Input: dimensioned drawing with shaded views. Units: mm. Origin: part minimum x, y, z. A direction names the side the tool comes from. Give positions to 0.01 mm unless a question says otherwise; leave off trailing zeros. Write each loop counter-clockwise with the first axis right and the second up, starting at its lowest first coordinate (ties: lowest second). Pieces come first, ordered by that corner, then holes. Notation, with made-up numbers: (3.25, -33) - (22.25, -33) arc R25 ccw to (22.25, 5) - close; hole circle Ø11 at (89, -4). An arc over 180 degrees is marked (long way). Answer as CSV lines item,"result".
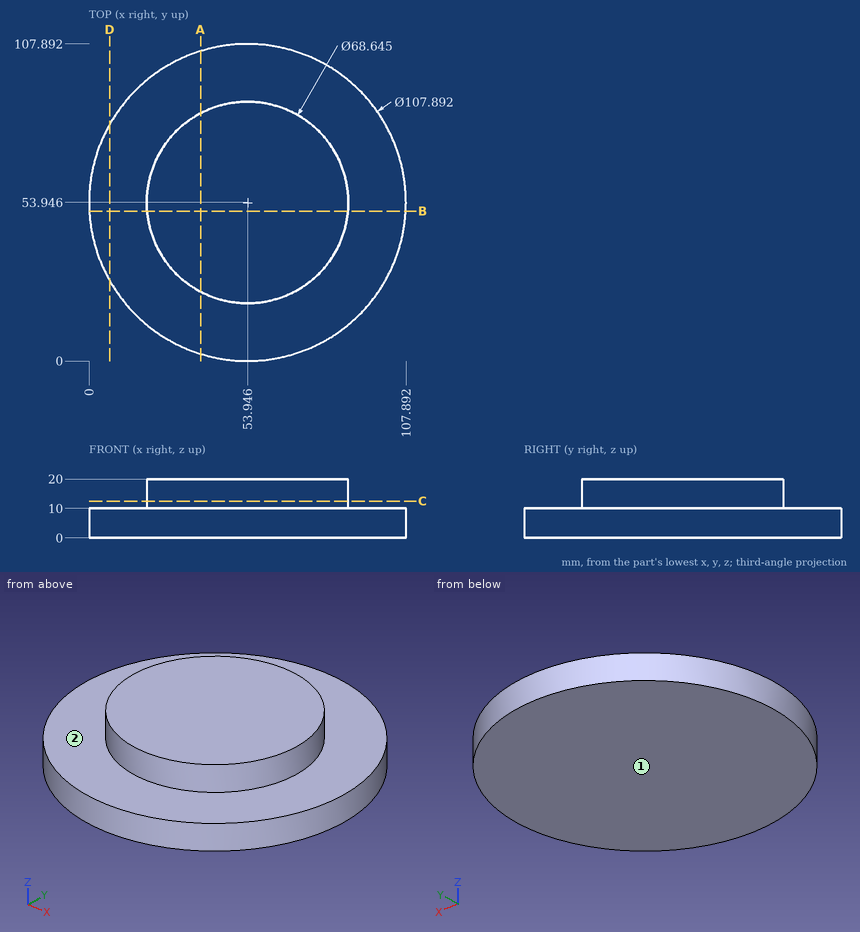
Item 1: Ray query, line 1 (Z direction, x = 82, y = 98.5); line 2 (X direction, y = 78, z = 15); line 3 (X direction, y = 24.5, z = 8.5) (1 decimal). Return the intervals inside material, ascending. Write a range as from..to.
The answers:
line 1,"0..10"
line 2,"29.46..78.43"
line 3,"8.7..99.1"
Item 2: Contact query for flat-ended pins moving along their axis: pin 1 (8 mm diameter, centred on y = 82, z = 14.5, fed in from -X); pin 2 (12 mm diameter, centred on x = 72.5, y = 84, fed in from -Z); pin 3 (5 mm diameter, centred on y = 48, z = 14.5, fed in from -X); pin 4 (6 mm diameter, centred on x = 56, z = 15.5, fed in from -Y). Output: stop coordinate, or through.
The answers:
pin 1,"x = 29.46"
pin 2,"z = 0"
pin 3,"x = 19.8"
pin 4,"y = 19.62"
Item 3: Reachability of the marked faces 1 and 2 from +Z, -Z, +X, -X, +Y, -Y: full face, straight path, thin tool, end or side. Return the list, or none.
The answers:
face 1,"-Z, +X, -X, +Y, -Y"
face 2,"+Z"
Item 4: Cut plane D-D on x = 7. Return the cut outline in (y, z).
The answers:
outline,"(27.37, 0) - (80.52, 0) - (80.52, 10) - (27.37, 10) - close"
Item 5: Cut plane C-C on z = 12.5. Return the cut outline in (x, y) (1 decimal).
The answers:
outline,"circle Ø68.6 at (53.9, 53.9)"
Item 6: Cut plane B-B on y = 51. Return the cut outline in (x, z).
The answers:
outline,"(0.08, 0) - (107.81, 0) - (107.81, 10) - (88.14, 10) - (88.14, 20) - (19.75, 20) - (19.75, 10) - (0.08, 10) - close"
Item 7: Cut plane A-A on x = 38. Return the cut outline in (y, z), plus the area to 3 significant figures.
The answers:
outline,"(2.41, 0) - (105.48, 0) - (105.48, 10) - (84.34, 10) - (84.34, 20) - (23.55, 20) - (23.55, 10) - (2.41, 10) - close"
area,"1,640 mm²"
